The drawing under review shows one solid part. Ordinate dimensions are in mm from its lowest x, y, z. Round coordinates to 2 decimals unless told otherwise and drop trailing zeros. Write each loop counter-clockwise with the first axis right and the second up, starting at its lowest first coordinate (ties: lowest second). Pieces come first, ordered by that corner, then holes. Notation, with made-up numbers: (20, 52.25) - (45, 52.25) arc R17 ccw to (45, 61.25) - close; hole circle Ø1 at (64, -37.5). An arc over 180 degrees is marked (long way). One line per question, with ' | ' between items. Start each with the question number.
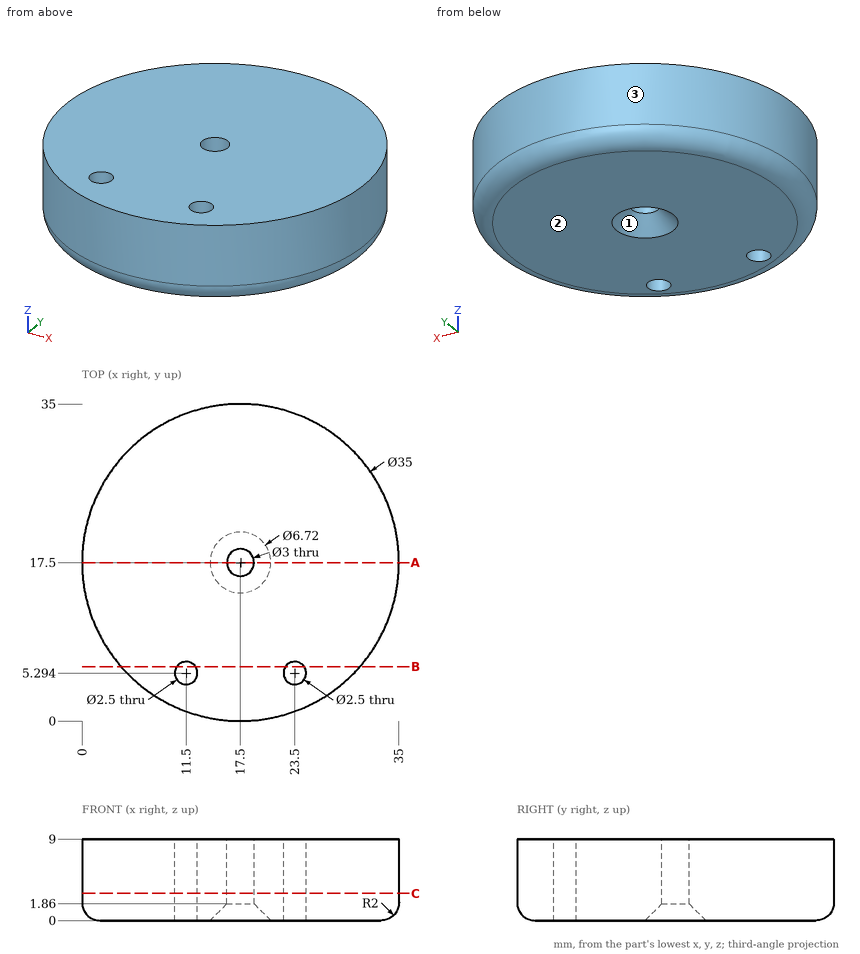
1. Clearance check with flat-ended pins moving along their axes: P1, Ø3, axis at x = 23.5, y = 5.29, coming from the +Z side; P2, Ø1.5, axis at y = 13, z = 4, coming from the +X side; P3, Ø2, axis at y = 22.5, z = 4.5, coming from the -X side; P4, Ø2.5, axis at x = 17.5, y = 17.5, coming from the -Z side. State where each tip first meets the part, or that it passes through.
2. Add section B-B, the plane y = 6. State how many separate pieces and enclosed holes the cut face has, then the cut area to 3 significant figures.
3. Wall thickness on line 1 along Y through (x, z) = (17.5, 4.5); line 2 along X through (y, z) = (18, 4.25) (1 decimal); line 3 along Y through (x, z) = (23.5, 4.5): over which ranges is each line inside the solid? List them lowest first. Write a range as [from, to].
4. Add section C-C, the plane z = 3. Write out the cut boundary in (x, y).
5. Add section A-A, the plane y = 17.5. Write out the cut boundary in (x, z), then the cut area to 3 significant figures.
6. The part is to be moulded in two halves that separate along X. For the marked faces 1, 2 and 3, say which applies: pulls with the +X half, pulls with the -X half, needs draft (parallel to the pull), parting line crosses it, or undercut.
Geometry check:
1) P1: stops at z = 9 | P2: stops at x = 34.59 | P3: stops at x = 0.46 | P4: passes through
2) separate pieces: 3 | enclosed holes: 0 | area: 198 mm2
3) line 1: y = [0, 16], [19, 35] | line 2: x = [0, 16.1], [18.9, 35] | line 3: y = [1.06, 4.04], [6.54, 33.94]
4) outline: circle Ø35 at (17.5, 17.5); hole circle Ø2.5 at (11.5, 5.29); hole circle Ø3 at (17.5, 17.5); hole circle Ø2.5 at (23.5, 5.29)
5) outline: (0, 2) arc R2 ccw to (2, 0) - (14.14, 0) - (16, 1.86) - (16, 9) - (0, 9) - close; (19, 1.86) - (20.86, 0) - (33, 0) arc R2 ccw to (35, 2) - (35, 9) - (19, 9) - close | area: 283 mm2
6) face 1: undercut | face 2: needs draft | face 3: parting line crosses it
